For this review, take the finished solid that the model builds, in its own axes (mm). Face numbers are marked on the shaded views. A direction names the side the tool comes from. Coordinates: 2 decimals unless noted, no trailing zeros. Write each loop counter-clockwise with the first axis right and the second up, starting at its lowest first coordinate (ties: lowest second). Pieces come first, ordered by that corner, then holes. Notation, with made-up numbers: M 81.5,-23.5 L 93.5,-23.5 A18 cw 93.5,-1.5 Z; hole C 10.25,48 d10. An arc over 180 degrees is marked long. Return JSON: item names as keys, results as strings.
```python
from build123d import *

# Parameters (mm, degrees)
F0_W      = 15
F0_H      = 80
F1_DEPTH  = 35
F2_W      = 15
F2_H      = 35
F3_DEPTH  = 50
F4_R      = 12.5
F5_DEPTH  = 5
F6_W      = 15
F6_H      = 35
F6_W_2    = 65
F7_DEPTH  = 15
F5_FACE_R = 12.5
F8_DEPTH  = 100


with BuildPart() as f1:
    # F0 (on Top) → F1 (new body)
    with BuildSketch(Plane.XY):
        with Locations((-45.405393, -2.018945)):
            Rectangle(F0_W, F0_H)
    extrude(amount=F1_DEPTH)

    # F2 (on face) → F3 (join)
    with BuildSketch(Plane.YZ.offset(-37.905393)):
        with Locations((30.481055, 17.5)):
            Rectangle(F2_W, F2_H)
    extrude(amount=F3_DEPTH)

    # F4 (on face) → F5 (cut)
    with BuildSketch(Plane.YZ.offset(-37.905393)):
        with Locations((-23.376025, 17.5)):
            Circle(F4_R)
        with Locations((7.423157, 17.5)):
            Circle(F4_R)
    extrude(amount=-F5_DEPTH, mode=Mode.SUBTRACT)

    # F6 (on face) → F7 (join)
    with BuildSketch(Plane.YZ.offset(12.094607)):
        with Locations((30.481055, 17.5)):
            Rectangle(F6_W, F6_H)
        with Locations((-9.518945, 17.5)):
            Rectangle(F6_W_2, F6_H)
    extrude(amount=F7_DEPTH)

    # F5_face (on face) → F8 (cut)
    with BuildSketch(Plane(origin=(-42.905393, -23.376025, 17.5), x_dir=(0, 1, 0), z_dir=(1, 0, 0))):
        Circle(F5_FACE_R)
        with Locations((30.799183, 0)):
            Circle(F5_FACE_R)
    extrude(amount=F8_DEPTH, mode=Mode.SUBTRACT)


solid = f1.part
```
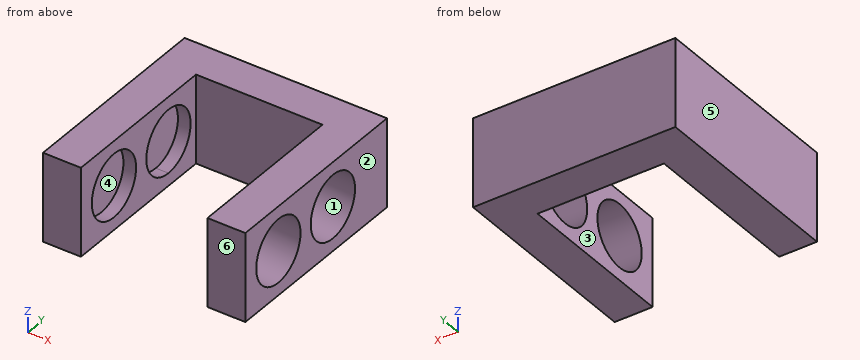
1. For the marked faces 1, 2 and 3, list the 3-axis set-ups (+Z, -Z, +X, -X, +Y, -Y) from which the entire face can be reached by the end or side of a thin tool; tool diameter is ignored.
Checks:
{"face 1": "+X", "face 2": "+Z, -Z, +X, +Y, -Y", "face 3": "+Z, -Z, -Y"}
2. Draft analysis for pull direction Y (two halves, no side actions). For the marked faces 4, 5 and 6, state which applies: +Y half, -Y half, draft (parallel to the pull), parting line (faces both ways), or undercut.
Checks:
{"face 4": "undercut", "face 5": "draft", "face 6": "-Y half"}
3. Wall thickness on L1, parallel to Y at x = 15.75, z = 17.5; L2, parallel to X at y = -14, z = 5; L3, parallel to Y at x = 19, z = 25: over which ranges is each line inside the solid? List them lowest first. Write a range as from..to.
Checks:
{"L1": "-42.02..-35.88, -10.88..-5.08, 19.92..37.98", "L2": "-52.91..-37.91, 12.09..27.09", "L3": "-42.02..-33.38, -13.38..-2.58, 17.42..37.98"}
4. We need section B-B (y = -22). State the section outline as (x, z) points, plus the area to 3 significant figures.
Checks:
{"outline": "M -52.91,0 L -37.91,0 L -37.91,5.08 L -42.91,5.08 L -42.91,29.92 L -37.91,29.92 L -37.91,35 L -52.91,35 Z; M 12.09,0 L 27.09,0 L 27.09,5.08 L 12.09,5.08 Z; M 12.09,29.92 L 27.09,29.92 L 27.09,35 L 12.09,35 Z", "area": "553 mm2"}
5. We need section D-D (y = 10.5). State the section outline as (x, z) points.
Checks:
{"outline": "M -52.91,0 L -37.91,0 L -37.91,5.38 L -42.91,5.38 L -42.91,29.62 L -37.91,29.62 L -37.91,35 L -52.91,35 Z; M 12.09,0 L 27.09,0 L 27.09,5.38 L 12.09,5.38 Z; M 12.09,29.62 L 27.09,29.62 L 27.09,35 L 12.09,35 Z"}
6. We need section A-A (z = 17.5). State the section outline as (x, y) points.
Checks:
{"outline": "M -52.91,-42.02 L -37.91,-42.02 L -37.91,-35.88 L -42.91,-35.88 L -42.91,-10.88 L -37.91,-10.88 L -37.91,-5.08 L -42.91,-5.08 L -42.91,19.92 L -37.91,19.92 L -37.91,22.98 L 12.09,22.98 L 12.09,19.92 L 27.09,19.92 L 27.09,37.98 L -52.91,37.98 Z; M 12.09,-42.02 L 27.09,-42.02 L 27.09,-35.88 L 12.09,-35.88 Z; M 12.09,-10.88 L 27.09,-10.88 L 27.09,-5.08 L 12.09,-5.08 Z"}
7. Clearance check with flat-ended pins moving along their axes: pin 1 Ø3 at (x, z) = (7, 28.5) entering from -Y; pin 2 Ø7.5 at (y, z) = (13.5, 22) entering from +X. State where each tip first meets the part, or that it passes through.
Checks:
{"pin 1": "y = 22.98", "pin 2": "x = -42.91"}
8. We need section C-C (z = 4). State the section outline as (x, y) points.
Checks:
{"outline": "M -52.91,-42.02 L -37.91,-42.02 L -37.91,22.98 L 12.09,22.98 L 12.09,-42.02 L 27.09,-42.02 L 27.09,37.98 L -52.91,37.98 Z"}
